Verification items for the finished model (mm, model axes). Round coordinates to 2 decimals unless told otherwise and drop trailing zeros. Write each loop counter-clockwise with the first axis right and the second up, starting at its lowest first coordinate (ties: lowest second). Pieces come first, ordered by that corner, then holes. Notation, with made-up numbers: (-1, 7) -> (9, 7) arc R31 cw to (9, 42) -> close; hole circle Ø1 at (79.5, 64.25). An arc over 180 degrees is marked (long way). Answer as a JSON object with one key per item and string values. Group by question number.
(1) Scan line: L1, parallel to Y at x = 4, z = 1.1. Record every from-to range of solid material in increasing order. Write a range as from..to.
(2) Sectioned sample at A-A on x = 67.5. Record the cut outline in (y, z).
(3) Gauge pin test, flat end, axial feed: pin 1 Ø2.5 at (x, y) = (4, 64.5) entering from -Z. Record the tip position at first contact, or that the pin passes through.
(4) Sectioned sample at B-B on y = 4. Record the cut outline in (x, z).
(5) Draft check along Y on faces 1 (the face through (67.76, 62.517, 1.479)), 2 (the face through (3.74, 66.483, 1.479)), 3 (the face through (0, 34, 1)), 4 (the face through (35, 68.5, 1)). Enter one of: released by +Y, released by -Y, zero draft, split by the parting line, or undercut.
```python
from build123d import *

# Parameters (mm, degrees)
ESBO_O1_W                = 71.5
ESBO_O1_H                = 68.5
ESBO_O1_R                = 2
RESSALTO_EXTRUS_O1_DEPTH = 3
FILETE1_R                = 3


with BuildPart() as part:
    # Esboço1 → Ressalto-extrusão1 (new body)
    with BuildSketch(Plane.XY):
        with Locations((35.75, 34.25)):
            Rectangle(ESBO_O1_W, ESBO_O1_H)
        with Locations((4, 64.5)):
            Circle(ESBO_O1_R, mode=Mode.SUBTRACT)
        with Locations(Location((67.5, 64.5, 0), (0, 0, 180))):
            Circle(ESBO_O1_R, mode=Mode.SUBTRACT)
        with Locations((67.5, 4)):
            Circle(ESBO_O1_R, mode=Mode.SUBTRACT)
        with Locations(Location((4, 4, 0), (0, 0, 180))):
            Circle(ESBO_O1_R, mode=Mode.SUBTRACT)
    extrude(amount=RESSALTO_EXTRUS_O1_DEPTH)

    # Filete1
    filete1_edges = [part.edges().sort_by_distance(p)[0] for p in [
        (0, 68.5, 1.5),
        (71.5, 68.5, 1.5),
        (71.5, 0, 1.5),
        (0, 0, 1.5),
    ]]
    fillet(filete1_edges, radius=FILETE1_R)


solid = part.part
```
Computed values:
{
 "1": {"L1": "0..2, 6..62.5, 66.5..68.5"},
 "2": {"outline": "(0, 0) -> (2, 0) -> (2, 3) -> (0, 3) -> close; (6, 0) -> (62.5, 0) -> (62.5, 3) -> (6, 3) -> close; (66.5, 0) -> (68.5, 0) -> (68.5, 3) -> (66.5, 3) -> close"},
 "3": {"pin 1": "through"},
 "4": {"outline": "(0, 0) -> (2, 0) -> (2, 3) -> (0, 3) -> close; (6, 0) -> (65.5, 0) -> (65.5, 3) -> (6, 3) -> close; (69.5, 0) -> (71.5, 0) -> (71.5, 3) -> (69.5, 3) -> close"},
 "5": {"face 1": "undercut", "face 2": "undercut", "face 3": "zero draft", "face 4": "released by +Y"}
}
